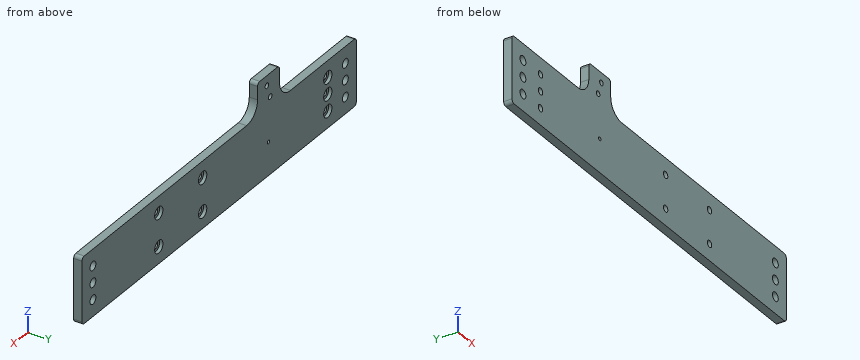
from build123d import *

# Parameters (mm, degrees)
SKETCH1_W                                       = 317.5
SKETCH1_H                                       = 50.8
BOSS_EXTRUDE1_DEPTH                             = 6.35
CBORE_FOR_10_SOCKET_HEAD_CAP_SCREW1_D           = 5.1054
CBORE_FOR_10_SOCKET_HEAD_CAP_SCREW1_CBORE_D     = 9.525
CBORE_FOR_10_SOCKET_HEAD_CAP_SCREW1_CBORE_DEPTH = 2.54
F_1_4_CLEARANCE_HOLE2_D                         = 6.7564
F_6_32_TAPPED_HOLE1_D                           = 2.7051
SKETCH12_W                                      = 25.4
SKETCH12_H                                      = 25.4
BOSS_EXTRUDE3_DEPTH                             = 6.35
F_10_32_TAPPED_HOLE1_D                          = 4.0386
FILLET1_R                                       = 12.7
FILLET2_R                                       = 2.54


with BuildPart() as part:
    # Sketch1 → Boss-Extrude1 (new body)
    with BuildSketch(Plane(origin=(0, 0, 0), x_dir=(1, 0, 0), z_dir=(0, 1, 0))):
        Rectangle(SKETCH1_W, SKETCH1_H)
    extrude(amount=BOSS_EXTRUDE1_DEPTH)

    # CBORE for #10 Socket Head Cap Screw1 (through all)
    with Locations(Plane(origin=(0, 6.35, 0), x_dir=(1, 0, 0), z_dir=(0, 1, 0))):
        with Locations((-125.73, -12.7), (19.05, 12.7), (69.85, 12.7), (19.05, -12.7), (69.85, -12.7), (-125.73, 12.7), (-125.73, 0)):
            CounterBoreHole(CBORE_FOR_10_SOCKET_HEAD_CAP_SCREW1_D / 2, CBORE_FOR_10_SOCKET_HEAD_CAP_SCREW1_CBORE_D / 2, CBORE_FOR_10_SOCKET_HEAD_CAP_SCREW1_CBORE_DEPTH)

    # 1/4 Clearance Hole2 (through all)
    with Locations(Plane.XZ):
        with Locations((-146.05, 12.7), (-146.05, 0), (-146.05, -12.7), (146.05, 12.7), (146.05, 0), (146.05, -12.7)):
            Hole(F_1_4_CLEARANCE_HOLE2_D / 2)

    # #6-32 Tapped Hole1 (through all)
    with Locations(Plane(origin=(0, 0, 0), x_dir=(-1, 0, 0), z_dir=(0, -1, 0))):
        with Locations((57.15, 0)):
            Hole(F_6_32_TAPPED_HOLE1_D / 2)

    # Sketch12 → Boss-Extrude3 (add)
    with BuildSketch(Plane(origin=(0, 6.35, 0), x_dir=(1, 0, 0), z_dir=(0, 1, 0))):
        with Locations((-57.15, -38.1)):
            Rectangle(SKETCH12_W, SKETCH12_H)
    extrude(amount=-BOSS_EXTRUDE3_DEPTH)

    # #10-32 Tapped Hole1 (through all)
    with Locations(Plane(origin=(0, 0, 0), x_dir=(-1, 0, 0), z_dir=(0, -1, 0))):
        with Locations((55.245, -43.18), (59.055, -33.02)):
            Hole(F_10_32_TAPPED_HOLE1_D / 2)

    # Fillet1
    fillet1_edges = [part.edges().sort_by_distance(p)[0] for p in [
        (-44.45, 3.175, 25.4),
        (-69.85, 3.175, 25.4),
    ]]
    fillet(fillet1_edges, radius=FILLET1_R)

    # Fillet2
    fillet2_edges = [part.edges().sort_by_distance(p)[0] for p in [
        (-44.45, 3.175, 50.8),
        (-69.85, 3.175, 50.8),
        (158.75, 3.175, 25.4),
        (-158.75, 3.175, 25.4),
        (-158.75, 3.175, -25.4),
        (158.75, 3.175, -25.4),
    ]]
    fillet(fillet2_edges, radius=FILLET2_R)


solid = part.part
For this review, take the finished solid that the model builds, in its own axes (mm). Give positions to 0.01 mm unless a question says otherwise; leave off trailing zeros. Write each loop counter-clockwise with the first axis right and the second up, starting at its lowest first coordinate (ties: lowest second). Pieces come first, ordered by that corner, then holes. Notation, with made-up numbers: (-4.75, -7.5) -> (8.25, -7.5) arc R23 ccw to (8.25, 18.5) -> close; hole circle Ø9 at (0.5, 36.5). An arc over 180 degrees is marked (long way). Use CSV: the item, a comma, the result in double quotes.
Q1. Take a section at D-D, the plane x = -41.5. Write out the cut boundary in (y, z).
Conclusion:
outline,"(0, -25.4) -> (6.35, -25.4) -> (6.35, 29.96) -> (0, 29.96) -> close"
Q2. For P1, Ø8.5, axis at x = 69.85, z = 12.7, coming from the +Y side; P2, Ø1.9, axis at y = 3.5, z = 43.5, coming from the +X side; P3, Ø1.5, axis at y = 2, z = 24, coming from the -X side, all flat-tipped, find the tip position at first contact; note any pin that passes through.
Conclusion:
P1,"y = 3.81"
P2,"x = -44.45"
P3,"x = -158.72"
Q3. Take a section at A-A, the plane x = -146.05. Write out the cut boundary in (y, z).
Conclusion:
outline,"(0, -25.4) -> (6.35, -25.4) -> (6.35, -16.08) -> (0, -16.08) -> close; (0, -9.32) -> (6.35, -9.32) -> (6.35, -3.38) -> (0, -3.38) -> close; (0, 3.38) -> (6.35, 3.38) -> (6.35, 9.32) -> (0, 9.32) -> close; (0, 16.08) -> (6.35, 16.08) -> (6.35, 25.4) -> (0, 25.4) -> close"
Q4. Take a section at C-C, the plane x = 3. Write out the cut boundary in (y, z), then the cut area to 3 significant figures.
Conclusion:
outline,"(0, -25.4) -> (6.35, -25.4) -> (6.35, 25.4) -> (0, 25.4) -> close"
area,"323 mm2"
Q5. Take a section at B-B, the plane y = 2.5. State how many separate pieces and enclosed holes the cut face has, then the cut area to 3 significant figures.
Conclusion:
separate pieces,"1"
enclosed holes,"16"
area,"16,400 mm2"
Q6. To check wall thickness, follow probe 1 along Z at (x, y) = (69.85, 1.3); probe 2 along Z at (x, y) = (145.5, 4); probe 3 along Z at (x, y) = (-125.73, 2.1). State the ranges of each line that lie inside material, in increasing order. Write a range as [from, to].
Conclusion:
probe 1,"[-25.4, -15.25], [-10.15, 10.15], [15.25, 25.4]"
probe 2,"[-25.4, -16.03], [-9.37, -3.33], [3.33, 9.37], [16.03, 25.4]"
probe 3,"[-25.4, -15.25], [-10.15, -2.55], [2.55, 10.15], [15.25, 25.4]"
